Here's the drawing with two shaded views (mm, measured from the low corner). I have some questions. A direction names the side the tool comes from. Round coordinates to 2 decimals unless told otherwise and drop trailing zeros. Loops run counter-clockwise (first coordinate to the right, second up) from the corner with the lowest first, then second, coordinate; pieces in that order, holes last.
(1) Will these pins go through, and if not, where does the flat tip stop? pin 1 Ø6.5 at (y, z) = (109.5, 6.5) entering from -X; pin 2 Ø6.5 at (y, z) = (110.5, 4.5) entering from +X; pin 3 Ø17 at (x, y) = (92.14, 77.5) entering from -Z; pin 4 Ø2 at (x, y) = (43.5, 58) entering from +Z.
(2) Thinking about a two-plate mould opening in Y: for the marked faces 1, 2 and 3, which applies, released by +Y, released by -Y, zero draft, split by the parting line, or undercut?
(3) I want a section at A-A on x = 57.5. Write out the boundary of the cut face in (y, z), plus the area to 3 significant figures.
(4) I want a section at B-B on z = 6.5. Write out the boundary of the cut face in (x, y).
(5) If I drill on line 1 along Y through (x, z) = (16, 6.5) (1 decimal); line 2 along Y through (x, z) = (53.5, 5.75) (1 decimal); line 3 along Y through (x, z) = (89, 8) (1 decimal), over which ranges is the centre line in solid material (lowest first)?
(6) Which directions (+Z, -Z, +X, -X, +Y, -Y) give clear straight access to the entire face, cutting with the end or side of a thin tool? Please do the marked faces 4, 5 and 6.
(7) I want a section at D-D on y = 48.5. Write out the boundary of the cut face in (x, z), plus the area to 3 significant figures.
(8) I want a section at C-C on y = 77.5. Write out the boundary of the cut face in (x, z), plus the area to 3 significant figures.
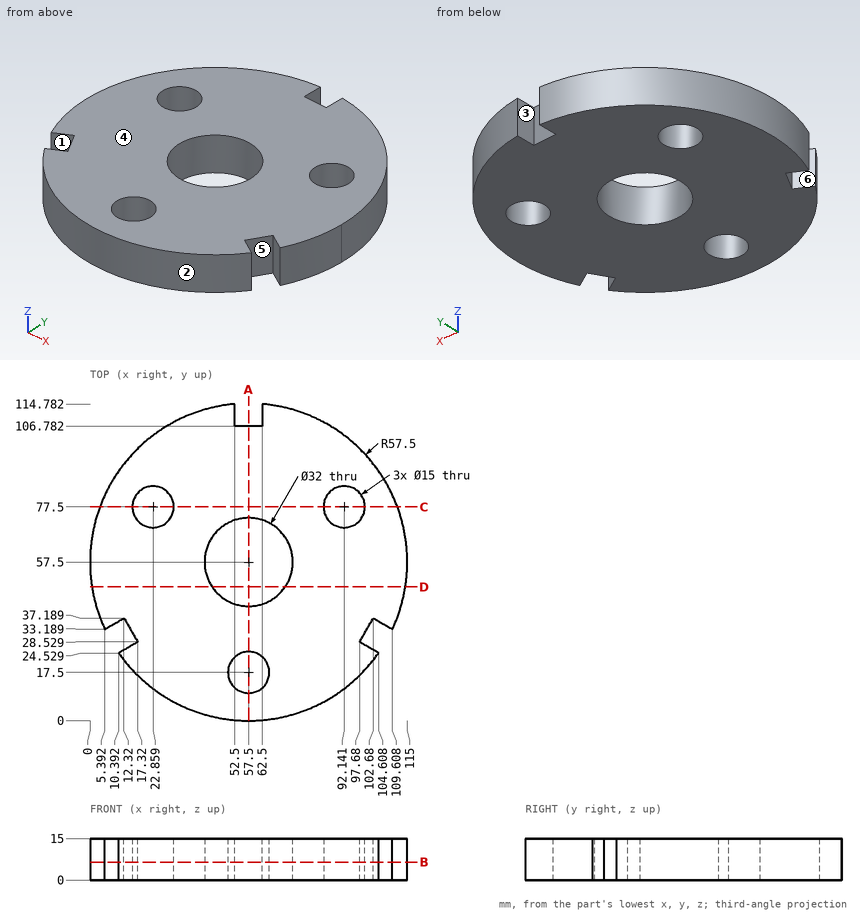
Filled sheet:
1. pin 1: stops at x = 27.01
1. pin 2: stops at x = 86.33
1. pin 3: stops at z = 0
1. pin 4: passes through
2. face 1: undercut
2. face 2: released by -Y
2. face 3: zero draft
3. outline: (0, 0) - (10, 0) - (10, 15) - (0, 15) - close; (25, 0) - (41.5, 0) - (41.5, 15) - (25, 15) - close; (73.5, 0) - (106.78, 0) - (106.78, 15) - (73.5, 15) - close
3. area: 897 mm2
4. outline: (5.39, 33.19) - (12.32, 37.19) - (17.32, 28.53) - (10.39, 24.53) arc R57.5 ccw to (104.61, 24.53) - (97.68, 28.53) - (102.68, 37.19) - (109.61, 33.19) arc R57.5 ccw to (62.5, 114.78) - (62.5, 106.78) - (52.5, 106.78) - (52.5, 114.78) arc R57.5 ccw to start; hole circle Ø15 at (22.86, 77.5); hole circle Ø32 at (57.5, 57.5); hole circle Ø15 at (57.5, 17.5); hole circle Ø15 at (92.14, 77.5)
5. line 1: y = 17.7 to 27.8, 30.8 to 74.5, 80.5 to 97.3
5. line 2: y = 0.1 to 11.2, 23.8 to 42, 73 to 106.8
5. line 3: y = 9.4 to 70.7, 84.3 to 105.6
6. face 4: +Z, +X, -X, +Y, -Y
6. face 5: +Z, -Z
6. face 6: +Z, -Z, -X
7. outline: (0.71, 0) - (44.27, 0) - (44.27, 15) - (0.71, 15) - close; (70.73, 0) - (114.29, 0) - (114.29, 15) - (70.73, 15) - close
7. area: 1,310 mm2
8. outline: (3.59, 0) - (15.36, 0) - (15.36, 15) - (3.59, 15) - close; (30.36, 0) - (84.64, 0) - (84.64, 15) - (30.36, 15) - close; (99.64, 0) - (111.41, 0) - (111.41, 15) - (99.64, 15) - close
8. area: 1,170 mm2
